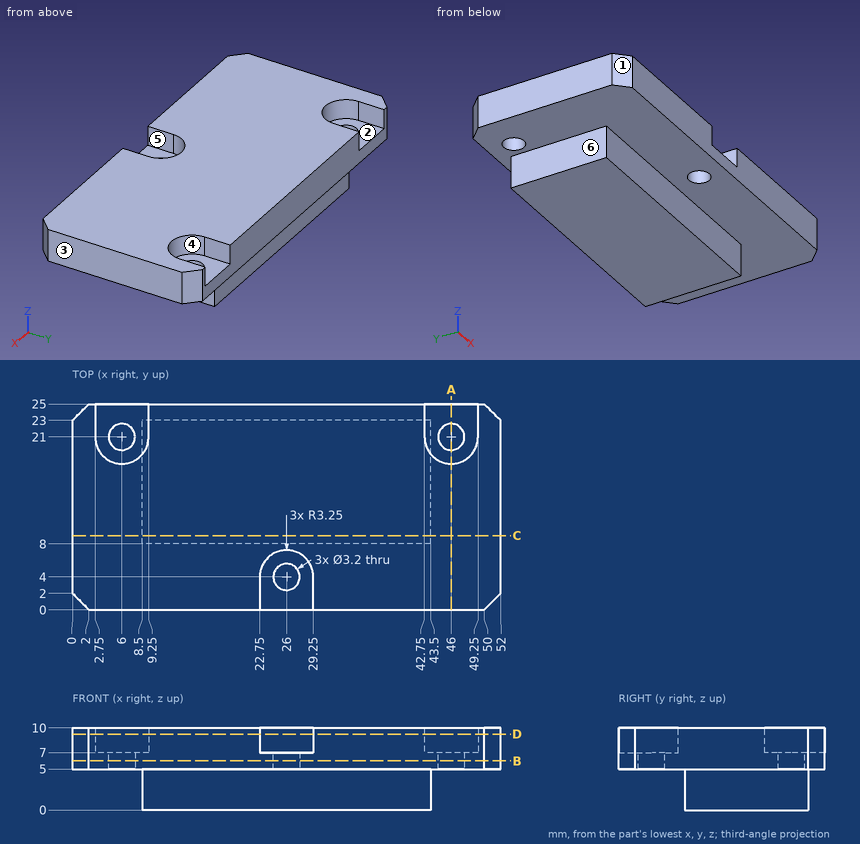
Geometry: see drawing. Coordinates: mm, zero at the bounding-box minimum. A direction names the side the tool comes from. Round coordinates to 2 decimals unless told otherwise and drop trailing zeros. Order: outer loops, then holes, each group sorted by start corner. A loop starts at its lowest first (then second) coordinate and runs counter-clockwise, first axis right, second up. Notation, with made-up numbers: (59.5, 5) - (83.5, 5) arc R9 cw to (83.5, 13) - close; hole circle Ø11 at (31, -39.5). An arc over 180 degrees is marked (long way). Use a Markdown table: item, result. Add a question column.
1. Section query B-B (z = 6). Return the cut outline in (x, y).
2. Section query D-D (z = 9.25). Return the cut outline in (x, y).
3. Section query A-A (x = 46). Return the cut outline in (y, z).
4. Section query C-C (y = 9). Return the cut outline in (x, z).
5. Mould query, pull axis X, two halves, no side actions, for the marked faces 1, 2 and 3. Classes: +X half, -X half, draft (parallel to the pull), parting line (faces both ways), or undercut.
6. Set-up query: the marked faces 4, 5 and 6. Return all of +Z, -Z, +X, -X, +Y, -Y with unobstructed straight access to the full face (end or side cutting, diameter ignored); none if empty.
7. First-contact query: pin 1 (1.5 mm diameter, centred on x = 20.5, z = 2.5, fed in from -Y); pin 2 (3 mm diameter, centred on x = 46, y = 20, fed in from +Z); pin 3 (2.5 mm diameter, centred on x = 6, y = 21, fed in from +Z); pin 4 (2.5 mm diameter, centred on y = 18, z = 3, fed in from +X). Flat tips, straight axial feed; report the tip coordinate or a pass-through.
8. Line query: probe 1 along X at (y, z) = (22.25, 8); probe 2 along X at (y, z) = (18.75, 8); probe 3 along Y at (x, z) = (6, 5.85). Output: solid intervals per line, ascending.
Derived:
| question | item | result |
|---|---|---|
| 1 | outline | (0, 2) - (2, 0) - (50, 0) - (52, 2) - (52, 23) - (50, 25) - (2, 25) - (0, 23) - close; hole circle Ø3.2 at (6, 21); hole circle Ø3.2 at (26, 4); hole circle Ø3.2 at (46, 21) |
| 2 | outline | (0, 2) - (2, 0) - (22.75, 0) - (22.75, 4) arc R3.25 cw to (29.25, 4) - (29.25, 0) - (50, 0) - (52, 2) - (52, 23) - (50, 25) - (49.25, 25) - (49.25, 21) arc R3.25 cw to (42.75, 21) - (42.75, 25) - (9.25, 25) - (9.25, 21) arc R3.25 cw to (2.75, 21) - (2.75, 25) - (2, 25) - (0, 23) - close |
| 3 | outline | (0, 5) - (19.4, 5) - (19.4, 7) - (17.75, 7) - (17.75, 10) - (0, 10) - close; (22.6, 5) - (25, 5) - (25, 7) - (22.6, 7) - close |
| 4 | outline | (0, 5) - (8.5, 5) - (8.5, 0) - (43.5, 0) - (43.5, 5) - (52, 5) - (52, 10) - (0, 10) - close |
| 5 | face 1 | -X half |
| 5 | face 2 | undercut |
| 5 | face 3 | +X half |
| 6 | face 4 | +Z, +Y |
| 6 | face 5 | +Z, -Y |
| 6 | face 6 | -Z, -X, +Y, -Y |
| 7 | pin 1 | y = 8 |
| 7 | pin 2 | z = 7 |
| 7 | pin 3 | through |
| 7 | pin 4 | x = 43.5 |
| 8 | probe 1 | 0 to 2.75, 9.25 to 42.75, 49.25 to 52 |
| 8 | probe 2 | 0 to 3.65, 8.35 to 43.65, 48.35 to 52 |
| 8 | probe 3 | 0 to 19.4, 22.6 to 25 |
